Can you work these out from the model? Positions are in its coordinate system, mm. Coordinates: 2 decimals unless noted, no trailing zeros. Loops run counter-clockwise (first coordinate to the right, second up) from the corner with the lowest first, then second, coordinate; pieces in that order, holes last.
```python
from build123d import *

# Parameters (mm, degrees)
FACE_PLATE_W           = 70
FACE_PLATE_H           = 110
FACE_PLATE_EXT_DEPTH   = 2
BUTTONS_R              = 6
BUTTONS_CUT_DEPTH      = 10
M3_TOP_SCREW_R         = 1.75
M3_TOP_SCREW_CUT_DEPTH = 10
FILLET1_R              = 2
FILLET2_R              = 2
FILLET3_R              = 2
FILLET4_R              = 2


with BuildPart() as part:
    # Face Plate → Face Plate Ext (new body)
    with BuildSketch(Plane(origin=(0, 0, 0), x_dir=(1, 0, 0), z_dir=(0, 1, 0))):
        Rectangle(FACE_PLATE_W, FACE_PLATE_H)
    extrude(amount=FACE_PLATE_EXT_DEPTH)

    # Buttons → Buttons CUT (cut)
    with BuildSketch(Plane(origin=(0, 2, 0), x_dir=(1, 0, 0), z_dir=(0, 1, 0))):
        with Locations(Location((-20, 30, 0), (0, 0, 270))):
            Circle(BUTTONS_R)
        with Locations(Location((15, 30, 0), (0, 0, 270))):
            Circle(BUTTONS_R)
        with Locations(Location((-20, 6.666666667, 0), (0, 0, 270))):
            Circle(BUTTONS_R)
        with Locations(Location((15, 6.666666667, 0), (0, 0, 270))):
            Circle(BUTTONS_R)
        with Locations(Location((-20, -16.666666667, 0), (0, 0, 270))):
            Circle(BUTTONS_R)
        with Locations(Location((-20, -40, 0), (0, 0, 270))):
            Circle(BUTTONS_R)
        with Locations(Location((15, -16.666666667, 0), (0, 0, 270))):
            Circle(BUTTONS_R)
        with Locations(Location((15, -40, 0), (0, 0, 270))):
            Circle(BUTTONS_R)
    extrude(amount=-BUTTONS_CUT_DEPTH, mode=Mode.SUBTRACT)

    # M3 Top Screw → M3 Top Screw CUT (cut)
    with BuildSketch(Plane(origin=(0, 2, 0), x_dir=(1, 0, 0), z_dir=(0, 1, 0))):
        with Locations(Location((-30, 50, 0), (0, 0, 270))):
            Circle(M3_TOP_SCREW_R)
        with Locations(Location((30, 50, 0), (0, 0, 270))):
            Circle(M3_TOP_SCREW_R)
        with Locations(Location((-30, -50, 0), (0, 0, 270))):
            Circle(M3_TOP_SCREW_R)
        with Locations(Location((30, -50, 0), (0, 0, 270))):
            Circle(M3_TOP_SCREW_R)
    extrude(amount=-M3_TOP_SCREW_CUT_DEPTH, mode=Mode.SUBTRACT)

    # M3 Head Top CUT cone 1 section (through the dimple's axis) → M3 Head Top CUT (revolve, cut)
    with BuildSketch(Plane(origin=(-30, 2, -50), x_dir=(0, 0, 1), z_dir=(1, 0, 0))):
        Polygon((0, 0), (2.8, 0), (0, 2.8), align=None)
    revolve(axis=Axis((-30, 2, -50), (0, -1, 0)), mode=Mode.SUBTRACT)

    # M3 Head Top CUT cone 2 section (through the dimple's axis) → M3 Head Top CUT cone 2 (revolve, cut)
    with BuildSketch(Plane(origin=(30, 2, -50), x_dir=(0, 0, 1), z_dir=(1, 0, 0))):
        Polygon((0, 0), (2.8, 0), (0, 2.8), align=None)
    revolve(axis=Axis((30, 2, -50), (0, -1, 0)), mode=Mode.SUBTRACT)

    # M3 Head Top CUT cone 3 section (through the dimple's axis) → M3 Head Top CUT cone 3 (revolve, cut)
    with BuildSketch(Plane(origin=(30, 2, 50), x_dir=(0, 0, 1), z_dir=(1, 0, 0))):
        Polygon((0, 0), (2.8, 0), (0, 2.8), align=None)
    revolve(axis=Axis((30, 2, 50), (0, -1, 0)), mode=Mode.SUBTRACT)

    # M3 Head Top CUT cone 4 section (through the dimple's axis) → M3 Head Top CUT cone 4 (revolve, cut)
    with BuildSketch(Plane(origin=(-30, 2, 50), x_dir=(0, 0, 1), z_dir=(1, 0, 0))):
        Polygon((0, 0), (2.8, 0), (0, 2.8), align=None)
    revolve(axis=Axis((-30, 2, 50), (0, -1, 0)), mode=Mode.SUBTRACT)

    # Fillet1
    fillet1_edges = [part.edges().sort_by_distance(p)[0] for p in [
        (-35, 1, -55),
    ]]
    fillet(fillet1_edges, radius=FILLET1_R)

    # Fillet2
    fillet2_edges = [part.edges().sort_by_distance(p)[0] for p in [
        (35, 1, -55),
    ]]
    fillet(fillet2_edges, radius=FILLET2_R)

    # Fillet3
    fillet3_edges = [part.edges().sort_by_distance(p)[0] for p in [
        (35, 1, 55),
    ]]
    fillet(fillet3_edges, radius=FILLET3_R)

    # Fillet4
    fillet4_edges = [part.edges().sort_by_distance(p)[0] for p in [
        (-35, 1, 55),
    ]]
    fillet(fillet4_edges, radius=FILLET4_R)


solid = part.part
```
Item 1: Suppose I cut it at B-B, the plane z = 40. Please give me the cut outline in (x, y), plus the area to 3 significant figures.
Results are:
outline: (-35, 0) - (-26, 0) - (-26, 2) - (-35, 2) - close; (-14, 0) - (9, 0) - (9, 2) - (-14, 2) - close; (21, 0) - (35, 0) - (35, 2) - (21, 2) - close
area: 92.0 mm2
Item 2: Suppose I cut it at C-C, the plane x = 15. Please give me the cut outline in (y, z), plus the area to 3 significant figures.
Results are:
outline: (0, -55) - (2, -55) - (2, -36) - (0, -36) - close; (0, -24) - (2, -24) - (2, -12.67) - (0, -12.67) - close; (0, -0.67) - (2, -0.67) - (2, 10.67) - (0, 10.67) - close; (0, 22.67) - (2, 22.67) - (2, 34) - (0, 34) - close; (0, 46) - (2, 46) - (2, 55) - (0, 55) - close
area: 124 mm2
Item 3: I need wall thicknesses on line 1 along X through (y, z) = (0.75, 50); line 2 along Z through (x, y) = (-19.5, 1); line 3 along X through (y, z) = (1.5, 40). Which ranges of each line are inside material? Lowest first, please.
Results are:
line 1: x = -35 to -31.75, -28.25 to 28.25, 31.75 to 35
line 2: z = -55 to -35.98, -24.02 to -12.65, -0.69 to 10.69, 22.65 to 34.02, 45.98 to 55
line 3: x = -35 to -26, -14 to 9, 21 to 35
Item 4: We'd pull the mould along Z, two halves only. Please class faces 1 (the face through (-15.945, 1.014, -11.089)), 2 (the face through (35, 1, 1)), 3 (the face through (34.4, 1.01, -54.43)): +Z half, -Z half, draft (parallel to the pull), parting line (faces both ways), or undercut.
Results are:
face 1: undercut
face 2: draft
face 3: -Z half
Item 5: I'm going to push flat-ended pins straight in: P1, Ø7, axis at x = -20, z = -6.67, coming from the +Y side; P2, Ø4.5, axis at x = 30, z = 50, coming from the +Y side. Where does each tip first touch, or does it pass through?
Results are:
P1: passes through
P2: stops at y = 1.45
Item 6: Suppose I cut it at A-A, the plane y = 0.5. Count the separate pieces of the cut face and the enclosed holes in it, plus the area to 3 significant figures.
Results are:
separate pieces: 1
enclosed holes: 12
area: 6,750 mm2
Item 7: Suppose I cut it at D-D, the plane x = 30. Please give me the cut outline in (y, z).
Results are:
outline: (0, -55) - (2, -55) - (2, -52.8) - (0.95, -51.75) - (0, -51.75) - close; (0, -48.25) - (0.95, -48.25) - (2, -47.2) - (2, 47.2) - (0.95, 48.25) - (0, 48.25) - close; (0, 51.75) - (0.95, 51.75) - (2, 52.8) - (2, 55) - (0, 55) - close
